```python
from build123d import *

# Parameters (mm, degrees)
BOSS_EXTRU_1_DEPTH           = 10
ENL_V_MAT_EXTRU_1_DEPTH      = 123.474487139
ENL_V_MAT_EXTRU_1_DEPTH_BACK = 123.474487139


with BuildPart() as part:
    # Esquisse1 → Boss.-Extru.1 (new body)
    with BuildSketch(Plane(origin=(0, 0, 0), x_dir=(1, 0, 0), z_dir=(0, 1, 0))):
        with BuildLine():
            Line((-100, 70), (-80, 70))
            ThreePointArc((-80, 70), (-68.284271247, 41.715728753), (-40, 30))
            Line((-40, 30), (40, 30))
            ThreePointArc((40, 30), (68.284271247, 41.715728753), (80, 70))
            Line((80, 70), (100, 70))
            ThreePointArc((100, 70), (83.475241575, 0), (100, -70))
            Line((100, -70), (80, -70))
            ThreePointArc((80, -70), (68.284271247, -41.715728753), (40, -30))
            Line((40, -30), (-40, -30))
            ThreePointArc((-40, -30), (-68.284271247, -41.715728753), (-80, -70))
            Line((-80, -70), (-100, -70))
            ThreePointArc((-100, -70), (-83.475241575, 0), (-100, 70))
        make_face()
        with BuildLine():
            Line((55, -20), (-55, -20))
            ThreePointArc((-55, -20), (-75, 0), (-55, 20))
            Line((-55, 20), (55, 20))
            ThreePointArc((55, 20), (75, 0), (55, -20))
        make_face(mode=Mode.SUBTRACT)
    extrude(amount=BOSS_EXTRU_1_DEPTH)

    # Esquisse2 → Enlèv. mat.-Extru.1 (cut, two sides: drawn at the far end of the back side and taken through both)
    with BuildSketch(Plane(origin=(0, 0, 0), x_dir=(0, 0, -1), z_dir=(1, 0, 0)).offset(-ENL_V_MAT_EXTRU_1_DEPTH_BACK)):
        with BuildLine():
            Line((70, 10), (0, 10))
            Line((0, 10), (0, 4.588098531))
            ThreePointArc((0, 4.588098531), (35.104446576, 5.943089657), (70, 10))
        make_face()
        with BuildLine():
            Line((0, 4.588098531), (0, 10))
            Line((0, 10), (-70, 10))
            ThreePointArc((-70, 10), (-35.104446576, 5.943089657), (0, 4.588098531))
        make_face()
        with BuildLine():
            Line((70, 10), (0, 10))
            Line((0, 10), (0, 4.588098531))
            ThreePointArc((0, 4.588098531), (35.104446576, 5.943089657), (70, 10))
        make_face()
        with BuildLine():
            Line((0, 4.588098531), (0, 10))
            Line((0, 10), (-70, 10))
            ThreePointArc((-70, 10), (-35.104446576, 5.943089657), (0, 4.588098531))
        make_face()
    extrude(amount=ENL_V_MAT_EXTRU_1_DEPTH + ENL_V_MAT_EXTRU_1_DEPTH_BACK, mode=Mode.SUBTRACT)


solid = part.part
```
Geometry: final body of the model. Coordinates: model frame, mm. A direction names the side the tool comes from. Give positions to 0.01 mm unless a question says otherwise; leave off trailing zeros. Loops run counter-clockwise (first coordinate to the right, second up) from the corner with the lowest first, then second, coordinate; pieces in that order, holes last. Notation, with made-up numbers: (29.5, 13) -> (52.5, 13) arc R19 cw to (52.5, 33) -> close; hole circle Ø2 at (-1.75, 39.25). An arc over 180 degrees is marked (long way). Use CSV: the item, a comma, the result in double quotes.
(1) Cut plane B-B (z = 60). Output: boundary loops of the cut face in (x, y), plus the area to 3 significant figures.
From the geometry:
outline,"(-95.43, 0) -> (-78.73, 0) -> (-78.73, 8.56) -> (-95.43, 8.56) -> close; (78.73, 0) -> (95.43, 0) -> (95.43, 8.56) -> (78.73, 8.56) -> close"
area,"286 mm^2"
(2) First-contact query: P1, Ø5, axis at x = 50.5, y = 7.5, coming from the -Z side; P2, Ø5, axis at y = 6, z = -22.5, coming from the -X side; P3, Ø3, axis at y = 1.5, z = 22.5, coming from the +X side. Flat tips, straight axial feed; report the tip coordinate or a pass-through.
From the geometry:
P1,"z = -31.92"
P2,"x = -85.47"
P3,"x = 85.33"
(3) Access query for faces 1 (the face through (1, 2, 20)), 2 (the face through (73.016, 3.819, 47.419)), 3 (the face through (-1, 3, -30)), 4 (the face through (-83.48, 3.82, 1.02)), 5 (the face through (83.48, 3.82, -1.02)). Directions: +Z, -Z, +X, -X, +Y, -Y. A direction counts if a zero-diameter tool reaches every point of the face in a straight line with its end or side. Return the directions, or none.
From the geometry:
face 1,"+Y, -Y"
face 2,"+Z, +Y, -Y"
face 3,"-Z, +Y, -Y"
face 4,"-X, +Y, -Y"
face 5,"+X, +Y, -Y"
(4) Pull-direction query (Z, two-part tool) for faces 6 (the face through (90, 5, 70)), 7 (the face through (75, 2, 0)), 8 (the face through (90, 5, -70)); classes: released by +Z, released by -Z, zero draft, split by the parting line, or undercut.
From the geometry:
face 6,"released by +Z"
face 7,"undercut"
face 8,"released by -Z"
(5) Cut plane A-A (x = 34). Output: boundary loops of the cut face in (y, z).
From the geometry:
outline,"(0, -30) -> (5.58, -30) arc R455.41 cw to (5.03, -20) -> (0, -20) -> close; (0, 20) -> (5.03, 20) arc R455.41 cw to (5.58, 30) -> (0, 30) -> close"
(6) Ray query, line 1 along Z through (x, y) = (-7, 4); line 2 along X through (y, z) = (1, -41.5); line 3 along Z through (x, y) = (-56.5, 0.5). Return the intervals inside material, ascending. Write a range as [from, to].
From the geometry:
line 1,"[-30, -20], [20, 30]"
line 2,"[-89.08, -68.07], [68.07, 89.08]"
line 3,"[-33.56, -19.94], [19.94, 33.56]"
(7) Cut plane C-C (x = -77). Output: boundary loops of the cut face in (y, z), plus the area to 3 significant figures.
From the geometry:
outline,"(0, -54.8) -> (7.9, -54.8) arc R455.41 cw to (7.9, 54.8) -> (0, 54.8) -> close"
area,"624 mm^2"
